from build123d import *

# Parameters (mm, degrees)
SKETCH2_W           = 8
SKETCH2_H           = 24
BOSS_EXTRUDE1_DEPTH = 3
SKETCH3_W           = 8
SKETCH3_H           = 3
BOSS_EXTRUDE2_DEPTH = 21
SKETCH7_R           = 1.75
CUT_EXTRUDE3_DEPTH  = 10
SKETCH8_R           = 1.75
CUT_EXTRUDE4_DEPTH  = 10


with BuildPart() as part:
    # Sketch2 → Boss-Extrude1 (new body)
    with BuildSketch(Plane.XY):
        with Locations((-53.564966099, 16.294171637)):
            Rectangle(SKETCH2_W, SKETCH2_H)
    extrude(amount=BOSS_EXTRUDE1_DEPTH)

    # Sketch3 → Boss-Extrude2 (add)
    with BuildSketch(Plane.XY.offset(3)):
        with Locations((-53.564966099, 5.794171637)):
            Rectangle(SKETCH3_W, SKETCH3_H)
    extrude(amount=BOSS_EXTRUDE2_DEPTH)

    # Sketch7 → Cut-Extrude3 (cut)
    with BuildSketch(Plane(origin=(0, 0, 0), x_dir=(-1, 0, 0), z_dir=(0, 0, -1))):
        with Locations((53.564966099, 12.294171637)):
            Circle(SKETCH7_R)
        with Locations((53.564966099, 20.294171637)):
            Circle(SKETCH7_R)
    extrude(amount=-CUT_EXTRUDE3_DEPTH, mode=Mode.SUBTRACT)

    # Sketch8 → Cut-Extrude4 (cut)
    with BuildSketch(Plane.XZ.offset(-4.294171637)):
        with Locations(Location((-53.564966099, 8, 0), (0, 0, 270))):
            Circle(SKETCH8_R)
        with Locations(Location((-53.564966099, 16, 0), (0, 0, 270))):
            Circle(SKETCH8_R)
    extrude(amount=-CUT_EXTRUDE4_DEPTH, mode=Mode.SUBTRACT)


solid = part.part
Here's how the part is built. I have some questions about the finished solid (model axes, mm). A direction names the side the tool comes from. Coordinates: 2 decimals unless noted, no trailing zeros. Write each loop counter-clockwise with the first axis right and the second up, starting at its lowest first coordinate (ties: lowest second). Pieces come first, ordered by that corner, then holes. Notation, with made-up numbers: (-32.75, -5.75) - (11.25, -5.75) arc R25 cw to (11.25, 24.25) - close; hole circle Ø9 at (56, 15.25). An arc over 180 degrees is marked (long way). Use one line per item in the form item = value.
1) Suppose I cut it at D-D, the plane y = 6.75. Write out the boundary of the cut face in (x, z), plus the area to 3 significant figures.
Solved:
outline = (-57.56, 0) - (-49.56, 0) - (-49.56, 24) - (-57.56, 24) - close; hole circle Ø3.5 at (-53.56, 8); hole circle Ø3.5 at (-53.56, 16)
area = 173 mm2
2) On a 3-axis mill with a long thin cutter (end or side, diameter ignored), from which of +Z, -Z, +X, -X, +Y, -Y can I reach the whole of each face in a straight line? I mean faces 1 (the flat face through (-54, 7.294, 13)), 2 (the flat face through (-54, 6, 24)). Say none if no direction works.
Solved:
face_1 = +Z, +X, -X, +Y
face_2 = +Z, +X, -X, +Y, -Y
3) Suppose I cut it at A-A, the plane z = 8. Write out the boundary of the cut face in (x, y).
Solved:
outline = (-57.56, 4.29) - (-55.31, 4.29) - (-55.31, 7.29) - (-57.56, 7.29) - close; (-51.81, 4.29) - (-49.56, 4.29) - (-49.56, 7.29) - (-51.81, 7.29) - close
4) Suppose I cut it at C-C, the plane y = 20.75. Write out the boundary of the cut face in (x, z), plus the area to 3 significant figures.
Solved:
outline = (-57.56, 0) - (-55.25, 0) - (-55.25, 3) - (-57.56, 3) - close; (-51.88, 0) - (-49.56, 0) - (-49.56, 3) - (-51.88, 3) - close
area = 13.9 mm2
5) I need wall thicknesses on line 1 (X direction, y = 5.55, z = 16); line 2 (Y direction, x = -52.5, z = 2); line 3 (Y direction, x = -51.5, z = 5.5). Which ranges of each line are inside material? Lowest first, please.
Solved:
line_1 = -57.56 to -55.31, -51.81 to -49.56
line_2 = 4.29 to 10.91, 13.68 to 18.91, 21.68 to 28.29
line_3 = 4.29 to 7.29
6) Thinking about a two-plate mould opening in X: for faces 3 (the flat face through (-54, 4.294, 12)), 4 (the flat face through (-49.565, 6, 7)), 5 (the cylindrical face through (-53.04, 5.77, 14.33)), which applies, released by +X, released by -X, zero draft, split by the parting line, or undercut?
Solved:
face_3 = zero draft
face_4 = released by +X
face_5 = undercut
7) I'm going to push flat-ended pins straight in: P1, Ø4, axis at x = -54.5, z = 19, coming from the +Y side; P2, Ø1.5, axis at x = -54.5, y = 23.5, coming from the +Z side; P3, Ø3, axis at x = -53.5, y = 7, coming from the -Z side. Where does each tip first touch, or does it pass through?
Solved:
P1 = 7.29
P2 = 3
P3 = 0
8) Suppose I cut it at B-B, the plane x = -54.75. Write out the boundary of the cut face in (y, z).
Solved:
outline = (4.29, 0) - (11.01, 0) - (11.01, 3) - (7.29, 3) - (7.29, 6.71) - (4.29, 6.71) - close; (4.29, 9.29) - (7.29, 9.29) - (7.29, 14.71) - (4.29, 14.71) - close; (4.29, 17.29) - (7.29, 17.29) - (7.29, 24) - (4.29, 24) - close; (13.58, 0) - (19.01, 0) - (19.01, 3) - (13.58, 3) - close; (21.58, 0) - (28.29, 0) - (28.29, 3) - (21.58, 3) - close
